Work out the finished part from the listing and answer in its coordinate system (mm). Face numbers are marked on the shaded views. A direction names the side the tool comes from. Coordinates: 2 decimals unless noted, no trailing zeros. Order: outer loops, then holes, each group sorted by start corner. A loop starts at its lowest first (then second) coordinate and runs counter-clockwise, first axis right, second up. Notation, with made-up numbers: (51, 66.25) -> (72, 66.25) arc R21 ccw to (72, 95.25) -> close; hole circle Ø5 at (89.5, 57). An arc over 180 degrees is marked (long way). Answer as CSV lines item,"result". Start each with the question number.
Item 1: Each of these flat-tipped pins is pushed along its axis until it touches: pin 1 Ø4.5 at (x, z) = (2.5, -1) entering from -Y; pin 2 Ø2 at (y, z) = (6.5, -1.5) entering from +X; pin 3 Ø3 at (y, z) = (6.5, 4) entering from -X; pin 4 Ø6.5 at (x, z) = (0, 0) entering from +Y. Where does it stop, or does it pass through?
Item 2: Straight lines are drawn through the part: L1, parallel to X at y = 1.5, z = 0; L2, parallel to Y at x = -4.25, z = 0.5; L3, parallel to Z at x = -4.5, y = 1.5. For each, find the intervals that lie inside material, in ascending order.
Item 3: For a pull along Z with two mould halves and no side action, classify the marked faces 1, 2 and 3 as pulls with the +Z half, pulls with the -Z half, needs draft (parallel to the pull), parting line crosses it, or undercut.
Item 4: Section A-A (y = 6.5) is taken. Write down the section's boundary in (x, z), then the cut area to 3 significant figures.
Item 5: Which of the six approach directions +Z, -Z, +X, -X, +Y, -Y give full straight-line access (tool end or side, diameter ignored) to the marked faces 4 and 5?
```python
from build123d import *

# Parameters (mm, degrees)
SKETCH_1_R          = 7.25
EXTRUDE_1_DEPTH     = 7.5
SKETCH_2_R          = 6.4
CUT_EXTRUDE_1_DEPTH = 6.3
SKETCH_4_R          = 4
CUT_EXTRUDE_2_DEPTH = 1.2
SKETCH_3_W          = 0.1
SKETCH_3_H          = 0.1


with BuildPart() as part:
    # ｽｹｯﾁ1 → ﾎﾞｽ - 押し出し1 (new body)
    with BuildSketch(Plane(origin=(0, 0, 0), x_dir=(1, 0, 0), z_dir=(0, 1, 0))):
        with Locations(Location((0, 0, 0), (0, 0, 270))):
            Circle(SKETCH_1_R)
    extrude(amount=EXTRUDE_1_DEPTH)

    # ｽｹｯﾁ2 → ｶｯﾄ - 押し出し1 (cut)
    with BuildSketch(Plane.XZ):
        with Locations(Location((0, 0, 0), (0, 0, 270))):
            Circle(SKETCH_2_R)
    extrude(amount=-CUT_EXTRUDE_1_DEPTH, mode=Mode.SUBTRACT)

    # ｽｹｯﾁ4 → ｶｯﾄ - 押し出し2 (cut)
    with BuildSketch(Plane(origin=(0, 7.5, 0), x_dir=(1, 0, 0), z_dir=(0, 1, 0))):
        with Locations(Location((0, 0, 0), (0, 0, 270))):
            Circle(SKETCH_4_R)
    extrude(amount=-CUT_EXTRUDE_2_DEPTH, mode=Mode.SUBTRACT)

    # ｽｹｯﾁ3 → ｶｯﾄ - 回転1 (revolve, cut)
    with BuildSketch(Plane.XY):
        with Locations((-7.2, 5.45)):
            Rectangle(SKETCH_3_W, SKETCH_3_H)
        with Locations((-7.2, 3.75)):
            Rectangle(SKETCH_3_W, SKETCH_3_H)
        with Locations((-7.2, 2.05)):
            Rectangle(SKETCH_3_W, SKETCH_3_H)
    revolve(axis=Axis((0, 7.5, 0), (0, -1, 0)), mode=Mode.SUBTRACT)


solid = part.part
```
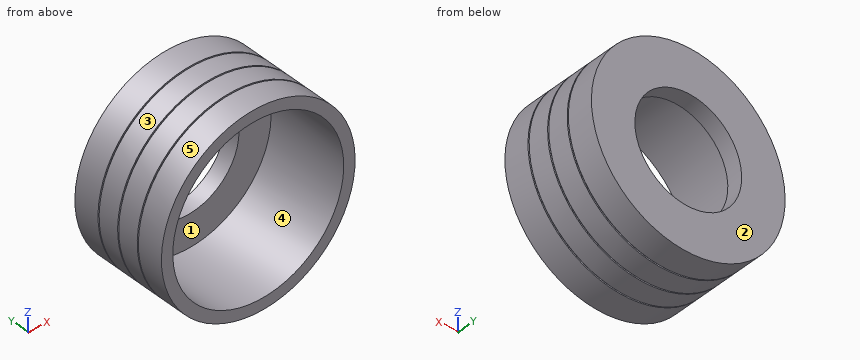
Checked values:
1,pin 1,"stops at y = 6.3"
1,pin 2,"stops at x = 7.23"
1,pin 3,"stops at x = -6.81"
1,pin 4,"passes through"
2,L1,"x = -7.25 to -6.4, 6.4 to 7.25"
2,L2,"y = 6.3 to 7.5"
2,L3,"z = -5.68 to -4.55, 4.55 to 5.68"
3,face 1,"undercut"
3,face 2,"needs draft"
3,face 3,"parting line crosses it"
4,outline,"circle Ø14.5 at (0, 0); hole circle Ø8 at (0, 0)"
4,area,"115 mm^2"
5,face 4,"-Y"
5,face 5,"+Y, -Y"
